Here's how the part is built. I have some questions about the finished solid (model axes, mm). Face numbers are marked on the shaded views. Round coordinates to 2 decimals unless told otherwise and drop trailing zeros. Write each loop counter-clockwise with the first axis right and the second up, starting at its lowest first coordinate (ties: lowest second). Pieces come first, ordered by that corner, then holes. Notation, with made-up numbers: (3, 8) - (55, 8) arc R12 ccw to (55, 21) - close; hole circle Ø2 at (37, -1). An arc over 180 degrees is marked (long way). Use one line per item in the form item = value. Start each with the question number.
1. We'd pull the mould along X, two halves only. Please class the marked faces 1, 2 and 3: +X half, -X half, draft (parallel to the pull), parting line (faces both ways), or undercut.
2. I want a section at A-A, the plane z = 3.25. List the corners of the cut face in (x, y) for me.
3. I want a section at B-B, the plane x = -12.5. List the corners of the cut face in (y, z) for me (3 decimals).
4. If I drill on line 1 along Z through (x, y) = (7.5, -11.5); line 2 along Y through (x, z) = (0.5, 0.5); line 3 along Z through (x, y) = (0, 0), over which ranges is the centre line in solid material (lowest first)?
5. Will these pins go through, and if not, where does the flat tip stop? pin 1 (6 mm diameter, centred on y = -2.5, z = 6.5, fed in from +X); pin 2 (1 mm diameter, centred on x = -3, y = -6.5, fed in from +Z); pin 3 (1 mm diameter, centred on y = -8, z = 7.5, fed in from -X).
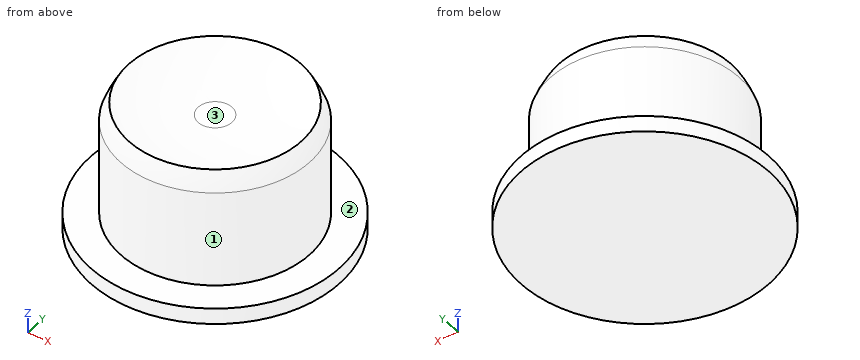
```python
from build123d import *


with BuildPart() as part:
    # Sketch → Revolution (revolve)
    with BuildSketch(Plane.XZ):
        with BuildLine():
            Line((0, 0), (-15.4, 0))
            Line((-15.4, 0), (-15.4, 2))
            Line((-15.4, 2), (-11.7, 2))
            Line((-11.7, 2), (-11.7, 14))
            ThreePointArc((-10.672007, 16.233973), (-11.24192, 15.142717), (-11.7, 14))
            ThreePointArc((-10.672007, 16.233973), (-6.459239, 15.049676), (-2.099769, 14.6689))
            Line((-2.099769, 14.6689), (0, 14.6689))
            Line((0, 14.6689), (0, 14))
            Line((0, 14), (0, 0))
        make_face()
    revolve(axis=Axis((0, 0, 0), (0, 0, 1)))


solid = part.part
```
Model answer:
q1.face_1 = parting line
q1.face_2 = draft
q1.face_3 = undercut
q2.outline = circle Ø23.4 at (0, 0)
q3.outline = (-8.995, 0) - (8.995, 0) - (8.995, 2) - (-8.995, 2) - close
q4.line_1 = 0 to 2
q4.line_2 = -15.39 to 15.39
q4.line_3 = 0 to 14.67
q5.pin_1 = 11.7
q5.pin_2 = 15.3
q5.pin_3 = -8.98
